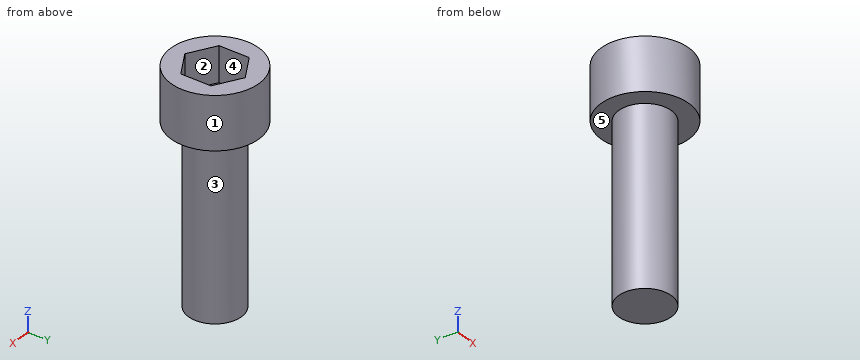
```python
from build123d import *

# Parameters (mm, degrees)
SKETCH_1_R          = 1.5
EXTRUDE_1_DEPTH     = 10
SKETCH_2_R          = 2.5
EXTRUDE_2_DEPTH     = 3
CUT_EXTRUDE_1_DEPTH = 2


with BuildPart() as part:
    # 草图1 → 凸台-拉伸1 (new body)
    with BuildSketch(Plane.XY):
        Circle(SKETCH_1_R)
    extrude(amount=EXTRUDE_1_DEPTH)

    # 草图2 → 凸台-拉伸2 (add)
    with BuildSketch(Plane.XY.offset(10)):
        Circle(SKETCH_2_R)
    extrude(amount=EXTRUDE_2_DEPTH)

    # 草图3 → 切除-拉伸1 (cut)
    with BuildSketch(Plane.XY.offset(13)):
        Polygon((0, 1.7), (-1.472243186, 0.85), (-1.472243186, -0.85), (0, -1.7), (1.472243186, -0.85), (1.472243186, 0.85), align=None)
    extrude(amount=-CUT_EXTRUDE_1_DEPTH, mode=Mode.SUBTRACT)


solid = part.part
```
Build history of the part. All positions in model axes, mm. Face numbers are marked on the shaded views. A direction names the side the tool comes from. Give positions to 0.01 mm unless a question says otherwise; leave off trailing zeros. Loops run counter-clockwise (first coordinate to the right, second up) from the corner with the lowest first, then second, coordinate; pieces in that order, holes last.
1) Two-plate mould, pull along Y, no slides. Class the marked faces 3, 4 and 5: released by +Y, released by -Y, zero draft, split by the parting line, or undercut.
Values follow:
face 3: split by the parting line
face 4: undercut
face 5: zero draft
2) Drop a flat-ended pin along its axis: P1, Ø1, axis at x = 1, z = 2, coming from the +Y side. Give the stop position or say it passes through.
Values follow:
P1: stops at y = 1.41
3) 3-axis set-ups, long thin cutter, end or side, ignore diameter. For the marked faces 1 and 2: which of +Z, -Z, +X, -X, +Y, -Y reach the whole face in a straight line?
Values follow:
face 1: +Z, -Z
face 2: +Z
4) Band-saw the part on C-C on z = 7.5. List the corners of the cut face in (x, y).
Values follow:
outline: circle Ø3 at (0, 0)
5) Band-saw the part on D-D on y = 1.85. List the corners of the cut face in (x, z), then the cut area to 3 significant figures.
Values follow:
outline: (-1.68, 10) - (1.68, 10) - (1.68, 13) - (-1.68, 13) - close
area: 10.1 mm2
6) Band-saw the part on B-B on x = -0.2. List the corners of the cut face in (y, z).
Values follow:
outline: (-2.49, 10) - (-1.49, 10) - (-1.49, 0) - (1.49, 0) - (1.49, 10) - (2.49, 10) - (2.49, 13) - (1.58, 13) - (1.58, 11) - (-1.58, 11) - (-1.58, 13) - (-2.49, 13) - close
7) Probe line 1 along Z through (x, y) = (1.2, 1.35); line 2 along Z through (x, y) = (-0.85, -0.45); line 3 along X through (y, z) = (-1.1, 11.5) (3 decimals). List the from-to ranges inside material, lowest first.
Values follow:
line 1: z = 10 to 13
line 2: z = 0 to 11
line 3: x = -2.245 to -1.039, 1.039 to 2.245
8) Band-saw the part on A-A on y = 0. List the corners of the cut face in (x, z).
Values follow:
outline: (-2.5, 10) - (-1.5, 10) - (-1.5, 0) - (1.5, 0) - (1.5, 10) - (2.5, 10) - (2.5, 13) - (1.47, 13) - (1.47, 11) - (-1.47, 11) - (-1.47, 13) - (-2.5, 13) - close
